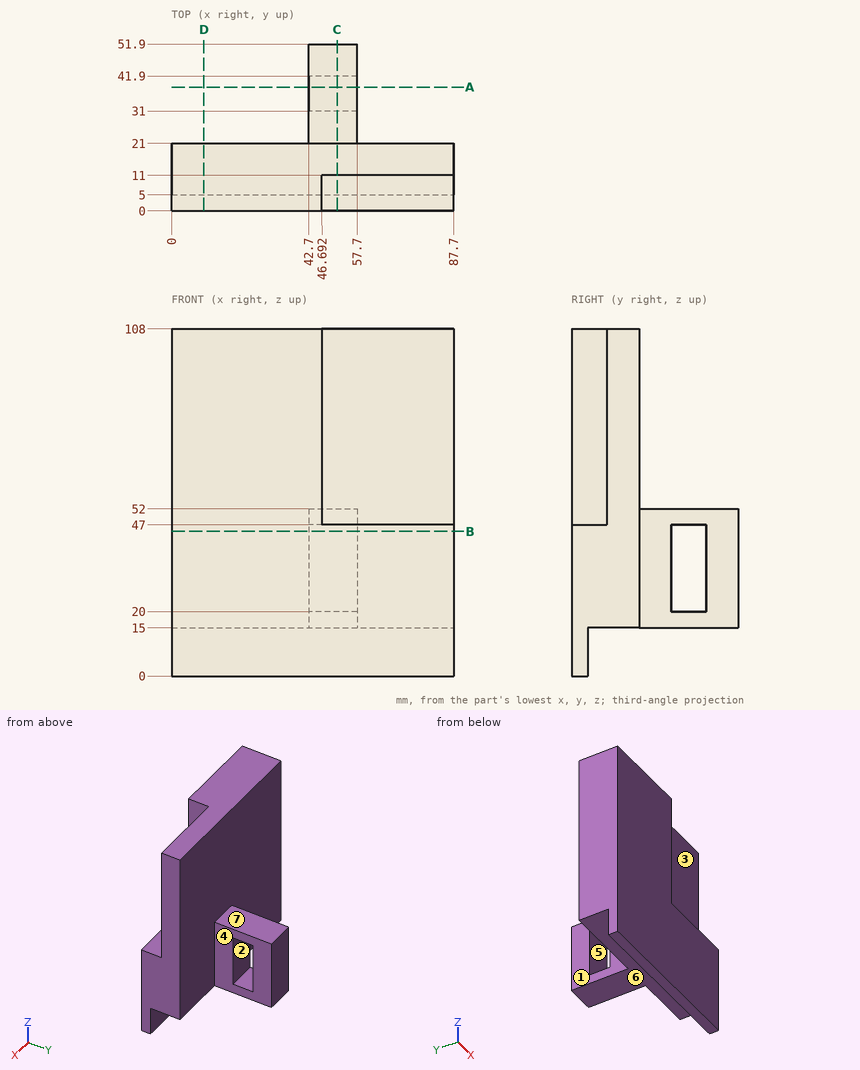
Input: dimensioned drawing with shaded views. Units: mm. Origin: part minimum x, y, z. A direction names the side the tool comes from. Round coordinates to 2 decimals unless told otherwise and drop trailing zeros. Order: outer loops, then holes, each group sorted by start corner. A loop starts at its lowest first (then second) coordinate and runs counter-clockwise, first axis right, second up. Notation, with made-up numbers: (21, 28) - (27, 28) arc R28 ccw to (27, 55) - close; hole circle Ø11 at (55, 20.5). An arc over 180 degrees is marked (long way). Answer as a JSON object with one key per item and string values. Group by question number.
(1) Cut plane A-A (y = 38.5). Return loops of the section in (x, z).
(2) Cut plane D-D (x = 10). Return loops of the section in (y, z).
(3) Cut plane C-C (x = 51.5). Return loops of the section in (y, z), then the cut area to 3 significant figures.
(4) Pin query (flat end, axial travel): P1, Ø8.5, axis at x = 49.5, y = 36, coming from the +Z side; P2, Ø4.5, axis at x = 50, z = 10.5, coming from the +Y side; P3, Ø9, axis at y = 4, z = 78.5, coming from the +X side. Return the tip coordinate at first contact, or that it passes through.
(5) Draft query along Y for the marked faces 1, 2 and 3. Return one class per face: released by +Y, released by -Y, zero draft, split by the parting line, or undercut.
(6) Material intervals for probe 1 along Y at (x, z) = (49, 24); probe 2 along Y at (x, z) = (32, 84.5); probe 3 along X at (y, z) = (36, 50), sorted ascending. Write a range as from..to.
(7) Cut plane B-B (z = 45). Return loops of the section in (x, y), then the cut area to 3 significant figures.
(8) Reachability of the marked faces 4, 5, 6 and 7 from +Z, -Z, +X, -X, +Y, -Y: full face, straight path, thin tool, end or side. Return the list, or none.
Here are the results:
{
 "1": {"outline": "(42.7, 15) - (57.7, 15) - (57.7, 20) - (42.7, 20) - close; (42.7, 47) - (57.7, 47) - (57.7, 52) - (42.7, 52) - close"},
 "2": {"outline": "(0, 0) - (5, 0) - (5, 15) - (21, 15) - (21, 108) - (0, 108) - close"},
 "3": {"outline": "(0, 0) - (5, 0) - (5, 15) - (51.9, 15) - (51.9, 52) - (21, 52) - (21, 108) - (11, 108) - (11, 47) - (0, 47) - close; hole (31, 20) - (41.9, 20) - (41.9, 47) - (31, 47) - close", "area": "2,210 mm^2"},
 "4": {"P1": "stops at z = 52", "P2": "stops at y = 5", "P3": "stops at x = 46.69"},
 "5": {"face 1": "zero draft", "face 2": "undercut", "face 3": "released by -Y"},
 "6": {"probe 1": "y = 0..31, 41.9..51.9", "probe 2": "y = 0..21", "probe 3": "x = 42.7..57.7"},
 "7": {"outline": "(0, 0) - (87.7, 0) - (87.7, 21) - (57.7, 21) - (57.7, 31) - (42.7, 31) - (42.7, 21) - (0, 21) - close; (42.7, 41.9) - (57.7, 41.9) - (57.7, 51.9) - (42.7, 51.9) - close", "area": "2,140 mm^2"},
 "8": {"face 4": "+Z, -Z, +X, +Y", "face 5": "+X, -X", "face 6": "-Z, +X, -X, +Y", "face 7": "+Z, +X, -X, +Y"}
}
